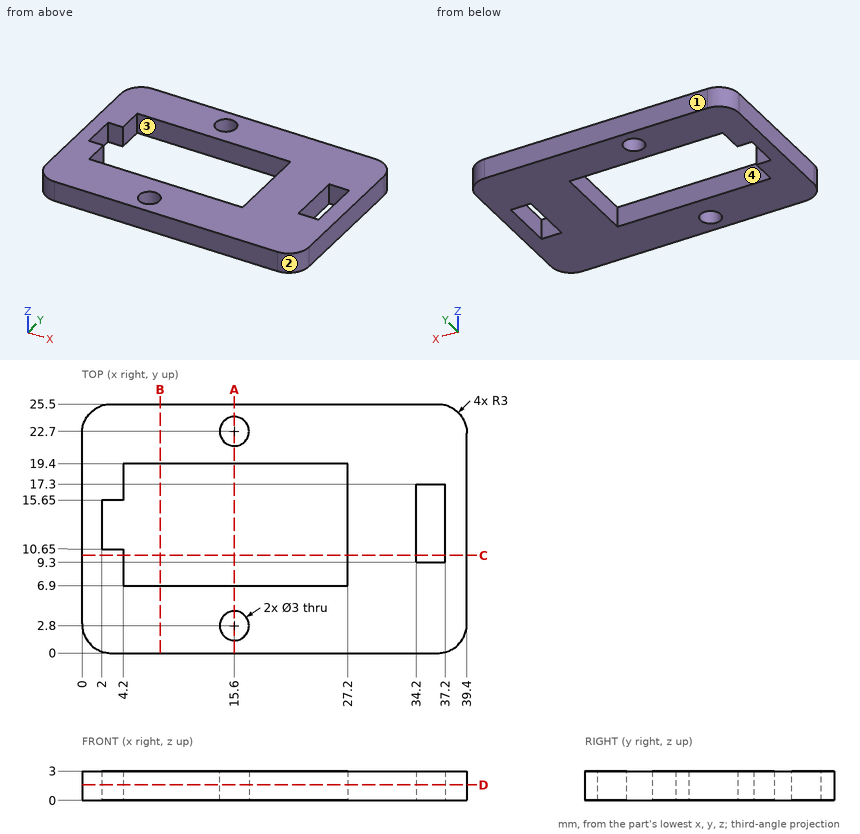
Job drawing, mm, ordinate dimensions from the low corner. One solid piece. Give positions to 0.01 mm unless a question says otherwise; leave off trailing zeros. Order: outer loops, then holes, each group sorted by start corner. A loop starts at its lowest first (then second) coordinate and runs counter-clockwise, first axis right, second up. Notation, with made-up numbers: (4, 71.5) -> (32, 71.5) arc R33 ccw to (32, 103.5) -> close; hole circle Ø4 at (-14, -27.75). An arc over 180 degrees is marked (long way). Return JSON: item names as keys, results as strings.
Q1. Saw through at D-D (z = 1.6). Write the cut outline in (x, y), then the cut area to 3 significant figures.
Working result:
{"outline": "(0, 3) arc R3 ccw to (3, 0) -> (36.4, 0) arc R3 ccw to (39.4, 3) -> (39.4, 22.5) arc R3 ccw to (36.4, 25.5) -> (3, 25.5) arc R3 ccw to (0, 22.5) -> close; hole (2, 10.65) -> (4.2, 10.65) -> (4.2, 6.9) -> (27.2, 6.9) -> (27.2, 19.4) -> (4.2, 19.4) -> (4.2, 15.65) -> (2, 15.65) -> close; hole circle Ø3 at (15.6, 2.8); hole circle Ø3 at (15.6, 22.7); hole (34.2, 9.3) -> (37.2, 9.3) -> (37.2, 17.3) -> (34.2, 17.3) -> close", "area": "660 mm²"}
Q2. Saw through at A-A (x = 15.6). Write the cut outline in (y, z).
Working result:
{"outline": "(0, 0) -> (1.3, 0) -> (1.3, 3) -> (0, 3) -> close; (4.3, 0) -> (6.9, 0) -> (6.9, 3) -> (4.3, 3) -> close; (19.4, 0) -> (21.2, 0) -> (21.2, 3) -> (19.4, 3) -> close; (24.2, 0) -> (25.5, 0) -> (25.5, 3) -> (24.2, 3) -> close"}
Q3. Mould opens along Y. For the marked faces 1, 2, 3 and 4 say: pulls with the +Y half, pulls with the -Y half, needs draft (parallel to the pull), parting line crosses it, or undercut.
Working result:
{"face 1": "pulls with the +Y half", "face 2": "pulls with the -Y half", "face 3": "undercut", "face 4": "undercut"}
Q4. Saw through at C-C (y = 10). Write the cut outline in (x, z).
Working result:
{"outline": "(0, 0) -> (4.2, 0) -> (4.2, 3) -> (0, 3) -> close; (27.2, 0) -> (34.2, 0) -> (34.2, 3) -> (27.2, 3) -> close; (37.2, 0) -> (39.4, 0) -> (39.4, 3) -> (37.2, 3) -> close"}
Q5. Saw through at B-B (x = 8). Write the cut outline in (y, z), then the cut area to 3 significant figures.
Working result:
{"outline": "(0, 0) -> (6.9, 0) -> (6.9, 3) -> (0, 3) -> close; (19.4, 0) -> (25.5, 0) -> (25.5, 3) -> (19.4, 3) -> close", "area": "39.0 mm²"}
Q6. Flat gauge pin, fed straight in: pin 1 (2.5 mm diameter, centred on x = 15.6, y = 2.8, fed in from -Z). Where does the tip first touch, or does it go through?
Working result:
{"pin 1": "through"}
Q7. Drill centre lines: line 1 (X direction, y = 12, z = 1.95); line 2 (Y direction, x = 15.6, z = 1.2); line 3 (X direction, y = 15.75, z = 2.2). Where is each one in solid material? Low to high.
Working result:
{"line 1": "0 to 2, 27.2 to 34.2, 37.2 to 39.4", "line 2": "0 to 1.3, 4.3 to 6.9, 19.4 to 21.2, 24.2 to 25.5", "line 3": "0 to 4.2, 27.2 to 34.2, 37.2 to 39.4"}
